For this review, take the finished solid that the model builds, in its own axes (mm). A direction names the side the tool comes from. Coordinates: 2 decimals unless noted, no trailing zeros. Loops run counter-clockwise (first coordinate to the right, second up) from the corner with the lowest first, then second, coordinate; pieces in that order, holes last. Notation, with made-up numbers: (76, -9.5) -> (113, -9.5) arc R9 cw to (113, -0.5) -> close; hole circle Ø10 at (-24.5, -38). An arc over 180 degrees is marked (long way). One line per item, written item: value.
from build123d import *

# Parameters (mm, degrees)
SKETCH1_W           = 100
SKETCH1_H           = 90
BOSS_EXTRUDE1_DEPTH = 2
SKETCH2_R           = 2.05
SKETCH2_R_2         = 2
BOSS_EXTRUDE3_DEPTH = 18.6
SKETCH2_5_R         = 1.25
CUT_EXTRUDE1_DEPTH  = 70.792263182
SKETCH2_6_R         = 1.2
BOSS_EXTRUDE4_DEPTH = 20.2
CUT_EXTRUDE2_DEPTH  = 2.2
LPATTERN1_COUNT     = 3
LPATTERN1_PITCH     = 22
SKETCH4_R           = 2
SKETCH4_R_2         = 2.05
BOSS_EXTRUDE5_DEPTH = 18.6
SKETCH4_3_R         = 1.25
CUT_EXTRUDE3_DEPTH  = 71.235603507
SKETCH4_4_R         = 1.2
BOSS_EXTRUDE6_DEPTH = 20.2
CUT_EXTRUDE4_DEPTH  = 2.2


with BuildPart() as part:
    # Sketch1 → Boss-Extrude1 (new, symmetric)
    with BuildSketch(Plane.XY):
        Rectangle(SKETCH1_W, SKETCH1_H)
    extrude(amount=BOSS_EXTRUDE1_DEPTH, both=True)

    # Sketch2 → Boss-Extrude3 (add)
    with BuildSketch(Plane.XY.offset(2)):
        with Locations((31.3, -18.68)):
            Circle(SKETCH2_R)
        with Locations((44, -18.68)):
            Circle(SKETCH2_R_2)
        with Locations((31.3, -39)):
            Circle(SKETCH2_R_2)
        with Locations((44, -39)):
            Circle(SKETCH2_R)
    boss_extrude3 = extrude(amount=-BOSS_EXTRUDE3_DEPTH)

    # Sketch2<5> → Cut-Extrude1 (cut, through all)
    with BuildSketch(Plane.XY.offset(2)):
        with Locations((44, -39)):
            Circle(SKETCH2_5_R)
        with Locations((31.3, -18.68)):
            Circle(SKETCH2_5_R)
    cut_extrude1 = extrude(amount=-CUT_EXTRUDE1_DEPTH, mode=Mode.SUBTRACT)

    # Sketch2<6> → Boss-Extrude4 (add)
    with BuildSketch(Plane.XY.offset(2)):
        with Locations((44, -18.68)):
            Circle(SKETCH2_6_R)
        with Locations((31.3, -39)):
            Circle(SKETCH2_6_R)
    boss_extrude4 = extrude(amount=-BOSS_EXTRUDE4_DEPTH)

    # Sketch3 → Cut-Extrude2 (cut)
    with BuildSketch(Plane.XY.offset(2)):
        Polygon((30.087564435, -16.58), (28.875128869, -18.68), (30.087564435, -20.78), (32.512435565, -20.78), (33.724871131, -18.68), (32.512435565, -16.58), align=None)
        Polygon((42.787564435, -36.9), (41.575128869, -39), (42.787564435, -41.1), (45.212435565, -41.1), (46.424871131, -39), (45.212435565, -36.9), align=None)
    cut_extrude2 = extrude(amount=-CUT_EXTRUDE2_DEPTH, mode=Mode.SUBTRACT)

    # LPattern1: Boss-Extrude3, Cut-Extrude1, Boss-Extrude4, Cut-Extrude2 ×3
    with Locations(*[(-i * LPATTERN1_PITCH, 0, 0) for i in range(1, LPATTERN1_COUNT)]):
        add(boss_extrude3)
        add(cut_extrude1, mode=Mode.SUBTRACT)
        add(boss_extrude4)
        add(cut_extrude2, mode=Mode.SUBTRACT)

    # Sketch4 → Boss-Extrude5 (add)
    with BuildSketch(Plane.XY.offset(2)):
        with Locations((-44, -39)):
            Circle(SKETCH4_R)
        with Locations((-26.22, -39)):
            Circle(SKETCH4_R_2)
        with Locations((-44, -18.68)):
            Circle(SKETCH4_R_2)
        with Locations((-26.22, -18.68)):
            Circle(SKETCH4_R)
    extrude(amount=-BOSS_EXTRUDE5_DEPTH)

    # Sketch4<3> → Cut-Extrude3 (cut, through all)
    with BuildSketch(Plane.XY.offset(2)):
        with Locations((-26.22, -39)):
            Circle(SKETCH4_3_R)
        with Locations((-44, -18.68)):
            Circle(SKETCH4_3_R)
    extrude(amount=-CUT_EXTRUDE3_DEPTH, mode=Mode.SUBTRACT)

    # Sketch4<4> → Boss-Extrude6 (add)
    with BuildSketch(Plane.XY.offset(2)):
        with Locations((-44, -39)):
            Circle(SKETCH4_4_R)
        with Locations((-26.22, -18.68)):
            Circle(SKETCH4_4_R)
    extrude(amount=-BOSS_EXTRUDE6_DEPTH)

    # Sketch5 → Cut-Extrude4 (cut)
    with BuildSketch(Plane.XY.offset(2)):
        Polygon((-45.212435565, -16.58), (-46.424871131, -18.68), (-45.212435565, -20.78), (-42.787564435, -20.78), (-41.575128869, -18.68), (-42.787564435, -16.58), align=None)
        Polygon((-27.432435565, -36.9), (-28.644871131, -39), (-27.432435565, -41.1), (-25.007564435, -41.1), (-23.795128869, -39), (-25.007564435, -36.9), align=None)
    extrude(amount=-CUT_EXTRUDE4_DEPTH, mode=Mode.SUBTRACT)


solid = part.part
1. Take a section at C-C, the plane y = 11.5. Give the boundary of the cut face in (x, z).
Return value:
outline: (-50, -2) -> (50, -2) -> (50, 2) -> (-50, 2) -> close
2. The part is to be moulded in two halves that separate along Y. For faces 4 (the cylindrical face through (9.95, -37.99, -17.39)), 5 (the flat face through (-1, -40, -16.6)), 6 (the cylindrical face through (43.01, -39.76, -8.29)), say which applies: pulls with the +Y half, pulls with the -Y half, needs draft (parallel to the pull), parting line crosses it, or undercut.
Return value:
face 4: parting line crosses it
face 5: needs draft
face 6: undercut
3. For faces 1 (the flat face through (-11, -39, -16.6)), 2 (the flat face through (0, -36.9, 1)), 3 (the flat face through (-14, -20, -16.6)), list the 3-axis set-ups (+Z, -Z, +X, -X, +Y, -Y) from which the entire face can be reached by the end or side of a thin tool; tool diameter is ignored.
Return value:
face 1: -Z
face 2: +Z
face 3: -Z, +Y
4. To check wall thickness, follow probe 1 along Y at (x, z) = (0, -5); probe 2 along Y at (x, z) = (31.3, -11.75); probe 3 along Y at (x, z) = (-12.5, 0.5). State the ranges of each line that lie inside material, in increasing order. Write a range as from..to.
Return value:
probe 1: y = -41.05..-40.25, -37.75..-36.95, -20.68..-16.68
probe 2: y = -41..-37, -20.73..-19.93, -17.43..-16.63
probe 3: y = -45..-20.78, -16.58..45
5. Take a section at A-A, the plane z = -13.5. Give the number of separate pieces and of enclosed holes in the cut face, and give its area (3 significant figures).
Return value:
separate pieces: 16
enclosed holes: 8
area: 167 mm2
6. Insertion check: pin 1 Ø2 at (x, y) = (44, -39) entering from -Z; pin 2 Ø3.5 at (x, y) = (31, -18) entering from -Z; pin 3 Ø10 at (x, z) = (-6.5, -15.5) entering from -Y; pin 4 Ø1.3 at (x, y) = (22, -38) entering from +Z. Each pin has a flat end and moves straight along its axis. Give the tip position at first contact, or say it passes through.
Return value:
pin 1: passes through
pin 2: stops at z = -16.6
pin 3: stops at y = -40.6
pin 4: stops at z = -0.2
7. Take a section at B-B, the plane x = -12.7. Give the boundary of the cut face in (y, z), and give its area (3 significant figures).
Return value:
outline: (-45, -2) -> (-41, -2) -> (-41, -16.6) -> (-40.2, -16.6) -> (-40.2, -18.2) -> (-37.8, -18.2) -> (-37.8, -16.6) -> (-37, -16.6) -> (-37, -2) -> (-20.73, -2) -> (-20.73, -16.6) -> (-19.93, -16.6) -> (-19.93, -0.2) -> (-20.78, -0.2) -> (-20.78, 2) -> (-45, 2) -> close; (-17.43, -16.6) -> (-16.63, -16.6) -> (-16.63, -2) -> (45, -2) -> (45, 2) -> (-16.58, 2) -> (-16.58, -0.2) -> (-17.43, -0.2) -> close
area: 432 mm2
8. Take a section at D-D, the plane x = -34. Give the boundary of the cut face in (y, z).
Return value:
outline: (-45, -2) -> (45, -2) -> (45, 2) -> (-45, 2) -> close
